Input: part model. Units: mm. Frame: model coordinates. Coordinates: 2 decimals unless noted, no trailing zeros. Loops run counter-clockwise (first coordinate to the right, second up) from the corner with the lowest first, then second, coordinate; pieces in that order, holes last. Notation, with made-up numbers: (42, 62) -> (57, 62) arc R13 cw to (57, 83) -> close; hole circle Ø4 at (-30.75, -18.75). An arc over 180 degrees is marked (long way). Answer as a JSON object with one key per item and string values.
Autodesk Inventor part; units mm, degrees
ref_plane "Work Plane1" through (-81.95, 0, 0) normal (-1, 0, 0) x (0, 0, 1)
ref_plane "YZ Plane" through (0, 0, 0) normal (1, 0, 0) x (0, 1, 0)
ref_plane "XZ Plane" through (0, 0, 0) normal (0, 1, 0) x (-1, 0, 0)
sketch "Sketch1" plane through (0, 0, 0) normal (0, 0, 1) x (1, 0, 0)
  line L0 (196.45, 0) -> (-196.45, 0)
  line L1 (-196.45, 0) -> (-196.45, 3.125)
  line L2 (-193.575, 6) -> (-193.5, 6)
  line L3 (-193.5, 6) -> (-193.5, 4)
  line L4 (-193.5, 4) -> (-189, 4)
  line L5 (-189, 4) -> (-189, 6)
  line L6 (-189, 6) -> (189, 6)
  line L7 (189, 6) -> (189, 4)
  line L8 (189, 4) -> (193.5, 4)
  line L9 (193.5, 4) -> (193.5, 6)
  line L10 (193.5, 6) -> (193.575, 6)
  line L11 (196.45, 3.125) -> (196.45, 0)
  arc A0 (-193.575, 6) -> (-196.45, 3.125) centre (-193.575, 3.125) ccw
  arc A1 (196.45, 3.125) -> (193.575, 6) centre (193.575, 3.125) ccw
  point P0 (0, 0)
  point P1 (0, 0)
  dimension "d2" = 12
  dimension "d4" = 8
  dimension "d5" = 12
  dimension "d7" = 8
  dimension "d8" = 12
  dimension "d15" = 2.875
  dimension "d21" = 2.95
  dimension "d22" = 4.5
  dimension "d23" = 2.95
  dimension "d24" = 4.5
  dimension "d29" = 387
revolve "Revolution1" add sketch "Sketch1" angle 360 about axis through (196.45, 0, 0) along (-1, 0, 0)
chamfer "Chamfer1" distance 2 angle 20 1 edges at (-189, -6, 0) measured on face at (-63, 5.9223, 0.9625)
fillet "Fillet1" radius 0.5 2 edges at (189, -4, 0) (-189, -4, 0)
chamfer "Chamfer2" distance 2 angle 20 1 edges at (189, -6, 0) measured on face at (-61.6667, 5.9805, 0.4828)
ref_plane "Work Plane1" through (-81.95, 0, 0) normal (-1, 0, 0) x (0, 0, 1)
split_face "Split1"
equation "\"d2\" = d5"
equation "\"d7\" = d4"
equation "\"d8\" = d5"
equation "\"d24\" = d22"
properties part number "311-03" material "Steel"
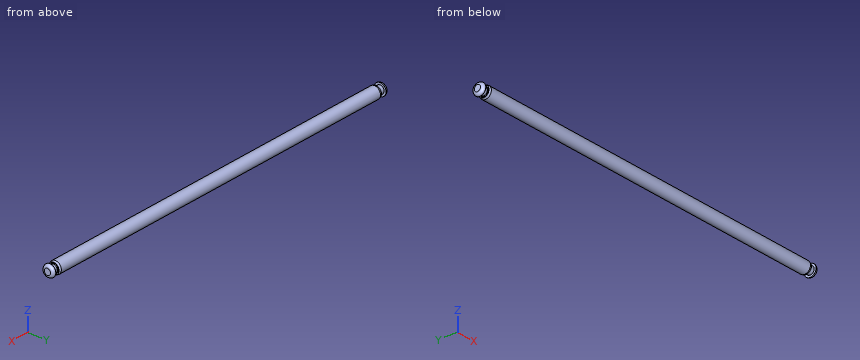
1. Section query A-A (x = -143). Return loops of the section in (y, z), plus the area to 3 significant figures.
Reply:
{"outline": "circle Ø12 at (0, 0)", "area": "113 mm2"}
2. Pin query (flat end, axial travel): P1, Ø6, axis at x = -110, z = 4, coming from the +Y side; P2, Ø1, axis at y = -4.5, z = -2.5, coming from the -X side; P3, Ø1.5, axis at y = -2, z = 4, coming from the +X side. Return the tip coordinate at first contact, or that it passes through.
Reply:
{"P1": "stops at y = 5.92", "P2": "stops at x = -196.01", "P3": "stops at x = 196.39"}
3. Line query: line 1 along X through (y, z) = (-3, 4.5); line 2 along X through (y, z) = (-4.5, -0.25); line 3 along Z through (x, y) = (73, -4.5). Output: solid intervals per line, ascending.
Reply:
{"line 1": "x = -195.32 to -193.5, -188.63 to 188.63, 193.5 to 195.32", "line 2": "x = -196.1 to -193.5, -189 to 189, 193.5 to 196.1", "line 3": "z = -3.97 to 3.97"}
